Read the model definition and answer for the solid it produces. Units are mm, in the model's axes. Face numbers are marked on the shaded views. Round coordinates to 2 decimals unless told otherwise and drop trailing zeros. Write each loop counter-clockwise with the first axis right and the second up, starting at its lowest first coordinate (ties: lowest second). Pieces come first, ordered by that corner, then holes. Notation, with made-up numbers: (12, 66.5) -> (37, 66.5) arc R15 ccw to (37, 86.5) -> close; hole circle Ø4 at (69.5, 58.5). An arc over 180 degrees is marked (long way). Return JSON: item names as keys, results as strings.
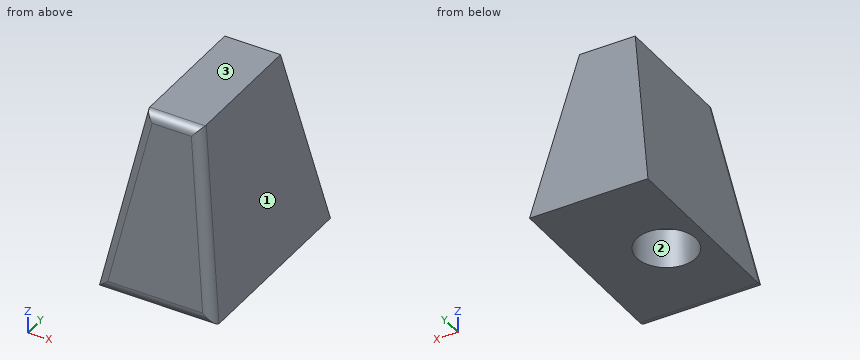
from build123d import *

# Parameters (mm, degrees)
F3_W     = 60
F3_H     = 100
F0_DEPTH = 90.0000035763
F0_TAPER = 10
F1_R     = 5
F2_R     = 15
F4_DEPTH = 20


with BuildPart() as f0:
    # F3 (on Top) → F0 (new body)
    with BuildSketch(Plane.XY):
        with Locations((30, 50)):
            Rectangle(F3_W, F3_H)
    extrude(amount=F0_DEPTH, taper=F0_TAPER)

    # F1
    f1_edges = [f0.edges().sort_by_distance(p)[0] for p in [
        (52.065286, 7.934714, 45.000002),
        (7.934714, 7.934714, 45.000002),
        (30, 0, 0),
        (30, 15.869429, 90.000004),
    ]]
    fillet(f1_edges, radius=F1_R)

    # F2 (on face) → F4 (cut)
    with BuildSketch(Plane(origin=(0, 0, 0), x_dir=(1, 0, 0), z_dir=(0, 0, -1))):
        with Locations((20.6221230328, -49.5650991797)):
            Circle(F2_R)
    extrude(amount=-F4_DEPTH, mode=Mode.SUBTRACT)


solid = f0.part
Item 1: Section D-D (y = 25) is taken. Give the vertices of the cut face in (x, z).
Worked answers:
{"outline": "(0, 0) -> (60, 0) -> (44.13, 90) -> (15.87, 90) -> close"}
Item 2: For a pull along X with two mould halves and no side action, classify the marked faces 1, 2 and 3 as released by +X, released by -X, zero draft, split by the parting line, or undercut.
Worked answers:
{"face 1": "released by +X", "face 2": "undercut", "face 3": "zero draft"}
Item 3: Section C-C (y = 52) is taken. Give the vertices of the cut face in (x, z), then the cut area to 3 significant figures.
Worked answers:
{"outline": "(0, 0) -> (5.82, 0) -> (5.82, 20) -> (35.42, 20) -> (35.42, 0) -> (60, 0) -> (44.13, 90) -> (15.87, 90) -> close", "area": "3,380 mm2"}
Item 4: Flat-ended cylindrical pins translate along their axes: pin 1 (10 mm diameter, centred on x = 15.5, z = 12, fed in from -Y); pin 2 (1 mm diameter, centred on x = 18, z = 76, fed in from +Y); pin 3 (15 mm diameter, centred on x = 22.5, y = 45.5, fed in from -Z). Find the tip coordinate at first contact, or state that the pin passes through.
Worked answers:
{"pin 1": "stops at y = 1.23", "pin 2": "stops at y = 86.69", "pin 3": "stops at z = 20"}
Item 5: Straight lines are drawn through the part: L1, parallel to Z at x = 23, y = 42; L2, parallel to X at y = 40, z = 4; L3, parallel to X at y = 26, z = 69.5. For each, find the intervals that lie inside material, in ascending order. Write a range as [from, to].
Worked answers:
{"L1": "z = [20, 90]", "L2": "x = [0.71, 9.07], [32.18, 59.29]", "L3": "x = [12.25, 47.75]"}
Item 6: Section B-B (x = 34) is taken. Give the vertices of the cut face in (y, z).
Worked answers:
{"outline": "(1.03, 5.87) arc R5 ccw to (5.96, 0) -> (42.78, 0) -> (42.78, 20) -> (56.35, 20) -> (56.35, 0) -> (100, 0) -> (84.13, 90) -> (20.06, 90) arc R5 ccw to (15.14, 85.87) -> close"}
Item 7: Section A-A (y = 40) is taken. Give the vertices of the cut face in (x, z), then the cut area to 3 significant figures.
Worked answers:
{"outline": "(0, 0) -> (9.07, 0) -> (9.07, 20) -> (32.18, 20) -> (32.18, 0) -> (60, 0) -> (44.13, 90) -> (15.87, 90) -> close", "area": "3,510 mm2"}
